Part model, mm, in its own coordinate system. A direction names the side the tool comes from. Coordinates: 2 decimals unless noted, no trailing zeros. Loops run counter-clockwise (first coordinate to the right, second up) from the corner with the lowest first, then second, coordinate; pieces in that order, holes last. Notation, with made-up numbers: M 53,49 L 67,49 A25 ccw 67,67 Z; hole C 40.5,5 d7. An arc over 180 degrees is marked long. Use a Markdown table: item, result. Add a question column.
1) Band-saw the part on A-A (x = 0). List the corners of the cut face in (y, z), plus the area to 3 significant figures.
2) Tool access for faces 5 (the flat face through (25, 0, -5)), 6 (the flat face through (4, 7, -3)), 7 (the flat face through (0, -20, -22)), 8 (the flat face through (-20, 0, -22)), 9 (the flat face through (0, -22, -10)): list every direction of +Z, -Z, +X, -X, +Y, -Y with a clear straight run to the whole face (end or side of a thin tool).
3) Band-saw the part on B-B (z = 337.5). List the corners of the cut face in (x, y), plus the area to 3 significant figures.
4) Pull direction X, two halves, no side cores. Call faces 1 (the flat face through (0, 20, -22)), 2 (the flat face through (25, 0, -40)), 3 (the flat face through (-25, 0, -40)), 4 (the flat face through (3, -10, -2)): released by +X, released by -X, zero draft, split by the parting line, or undercut.
5) Wall check: probe 1 along Y at (x, z) = (0, -1.1); probe 2 along Y at (x, z) = (0, -2.35); probe 3 along Z at (x, y) = (-23, 20.5). Give the ranges that are in metal, low to high. Write a range as from..to.
6) Pin check, flat tips, straight feed: pin 1 Ø12.5 at (y, z) = (3, -16.5) entering from +X; pin 2 Ø12 at (y, z) = (-5.5, 104) entering from -X; pin 3 Ø8 at (x, y) = (-15, -11.5) entering from +Z. Stop position of each tip, or through.
Autodesk Inventor part; units mm, degrees
ref_plane "YZ Plane" through (0, 0, 0) normal (1, 0, 0) x (0, 1, 0)
ref_plane "XZ Plane" through (0, 0, 0) normal (0, 1, 0) x (-1, 0, 0)
ref_plane "XY Plane" through (0, 0, 0) normal (0, 0, 1) x (1, 0, 0)
sketch "草图1" plane through (0, 0, 0) normal (0, 0, 1) x (1, 0, 0)
  circle A0 centre (0, 0) radius 4.25
  dimension "d0" = 8.5
extrude "拉伸1" add sketch "草图1" along normal blind 450
sketch "草图2" plane through (0, 0, 0) normal (0, 0, -1) x (-1, 0, 0)
  line L0 (-25, 25) -> (25, 25)
  line L1 (25, 25) -> (25, -25)
  line L2 (25, -25) -> (-25, -25)
  line L3 (-25, -25) -> (-25, 25)
  circle A0 centre (0, 0) radius 4.25
  line L4 (-25, 25) -> (25, -25) construction
  line L5 (25, 25) -> (-25, -25) construction
  dimension "d3" = 50
  dimension "d4" = 50
extrude "拉伸2" add sketch "草图2" along normal blind 10 contours L0 L1 L2 L3 | A0
sketch "草图3" plane through (0, 0, 0) normal (0, 0, 1) x (1, 0, 0)
  circle A0 centre (0, 0) radius 15
  dimension "d7" = 30
extrude "拉伸3" cut sketch "草图3" against normal blind 2
sketch "草图4" plane through (0, 0, -2) normal (0, 0, 1) x (1, 0, 0)
  circle A0 centre (0, 0) radius 10
  dimension "d10" = 20
extrude "拉伸4" cut sketch "草图4" against normal blind 1
sketch "草图5" plane through (0, 0, -3) normal (0, 0, 1) x (1, 0, 0)
  circle A0 centre (0, 0) radius 7.5
  dimension "d13" = 15
extrude "拉伸5" add sketch "草图5" along normal blind 2
sketch "草图6" plane through (0, 0, -1) normal (0, 0, 1) x (1, 0, 0)
  circle A0 centre (0, 0) radius 4.25
extrude "拉伸6" add sketch "草图6" along normal blind 2
sketch "草图7" plane through (0, 0, -10) normal (0, 0, -1) x (-1, 0, 0)
  line L0 (-20, 20) -> (20, 20)
  line L1 (20, 20) -> (20, -20)
  line L2 (20, -20) -> (-20, -20)
  line L3 (-20, -20) -> (-20, 20)
  line L4 (-20, 20) -> (20, -20) construction
  line L5 (20, 20) -> (-20, -20) construction
  point P0 (0, 0)
  dimension "d18" = 40
  dimension "d19" = 40
extrude "拉伸7" add sketch "草图7" along normal blind 25
sketch "草图8" plane through (0, 0, -35) normal (0, 0, -1) x (-1, 0, 0)
  line L0 (25, -25) -> (25, 25)
  line L1 (-25, 25) -> (25, 25)
  line L2 (25, 25) -> (25, -25)
  line L3 (25, -25) -> (-25, -25)
  line L4 (-25, -25) -> (-25, 25)
  circle A0 centre (0, 0) radius 7.5
  line L5 (-25, 25) -> (25, -25) construction
  line L6 (25, 25) -> (-25, -25) construction
  dimension "d22" = 50
  dimension "d23" = 50
extrude "拉伸8" add sketch "草图8" along normal blind 10 contours L3 L4 L1 L0 | A0
chamfer "倒角1" distance 5 angle 45 12 edges at (20, -20, -22.5) (25, -25, -5) (25, -25, -40) (-25, -25, -40) (-20, -20, -22.5) (-25, -25, -5) (25, 25, -5) (20, 20, -22.5) (25, 25, -40) (-20, 20, -22.5) (-25, 25, -5) (-25, 25, -40)
thread "螺纹1"
properties part number "步进电机"
Entries:
| question | item | result |
|---|---|---|
| 1 | outline | M -25,-45 L 25,-45 L 25,-35 L 20,-35 L 20,-10 L 25,-10 L 25,0 L 15,0 L 15,-2 L 10,-2 L 10,-3 L 7.5,-3 L 7.5,-1 L 4.25,-1 L 4.25,450 L -4.25,450 L -4.25,-1 L -7.5,-1 L -7.5,-3 L -10,-3 L -10,-2 L -15,-2 L -15,0 L -25,0 L -25,-10 L -20,-10 L -20,-35 L -25,-35 Z |
| 1 | area | 5,780 mm2 |
| 2 | face 5 | +Z, -Z, +X, +Y, -Y |
| 2 | face 6 | +Z |
| 2 | face 7 | +X, -X, -Y |
| 2 | face 8 | -X, +Y, -Y |
| 2 | face 9 | none |
| 3 | outline | C 0,0 d8.5 |
| 3 | area | 56.7 mm2 |
| 4 | face 1 | zero draft |
| 4 | face 2 | released by +X |
| 4 | face 3 | released by -X |
| 4 | face 4 | undercut |
| 5 | probe 1 | -25..-15, -7.5..7.5, 15..25 |
| 5 | probe 2 | -25..-10, -7.5..7.5, 10..25 |
| 5 | probe 3 | -45..-35, -10..0 |
| 6 | pin 1 | x = 20 |
| 6 | pin 2 | x = -4.25 |
| 6 | pin 3 | z = 0 |
